```python
from build123d import *

# Parameters (mm, degrees)
SKETCH1_R           = 6
SKETCH1_R_2         = 4.1
BOSS_EXTRUDE1_DEPTH = 5
SKETCH7_R           = 2.6
CUT_EXTRUDE1_DEPTH  = 7
BOSS_EXTRUDE7_DEPTH = 8
SKETCH9_R           = 1.6
CUT_EXTRUDE2_DEPTH  = 7
CUT_EXTRUDE3_DEPTH  = 10
SKETCH11_R          = 1
CUT_EXTRUDE4_DEPTH  = 10


with BuildPart() as part:
    # Sketch1 → Boss-Extrude1 (new body)
    with BuildSketch(Plane.XY):
        with BuildLine():
            Line((-58.265804598, 27.46480771), (50.206034483, 32.957769253))
            ThreePointArc((50.206034483, 32.957769253), (84.875, 0), (50.206034483, -32.957769253))
            Line((50.206034483, -32.957769253), (-58.265804598, -27.46480771))
            ThreePointArc((-58.265804598, -27.46480771), (-61.107119662, -27.172397082), (-63.902777778, -26.586845234))
            Line((-63.902777778, -26.586845234), (-105.963888889, -15.468709954))
            ThreePointArc((-105.963888889, -15.468709954), (-117.875, 0), (-105.963888889, 15.468709954))
            Line((-105.963888889, 15.468709954), (-63.902777778, 26.586845234))
            ThreePointArc((-63.902777778, 26.586845234), (-61.107119662, 27.172397082), (-58.265804598, 27.46480771))
        make_face()
        with Locations((51.875, 0)):
            Circle(SKETCH1_R, mode=Mode.SUBTRACT)
        with Locations((-101.875, 0)):
            Circle(SKETCH1_R_2, mode=Mode.SUBTRACT)
        with BuildLine():
            Line((-46.875, -18.2), (-56.875, -18.2))
            ThreePointArc((-56.875, -18.2), (-75.075, 0), (-56.875, 18.2))
            Line((-56.875, 18.2), (-46.875, 18.2))
            ThreePointArc((-46.875, 18.2), (-28.675, 0), (-46.875, -18.2))
        make_face(mode=Mode.SUBTRACT)
    extrude(amount=BOSS_EXTRUDE1_DEPTH)

    # Sketch7 → Cut-Extrude1 (cut)
    with BuildSketch(Plane.XY.offset(5)):
        with Locations((29.375, 0)):
            Circle(SKETCH7_R)
        with Locations((74.375, 0)):
            Circle(SKETCH7_R)
    extrude(amount=-CUT_EXTRUDE1_DEPTH, mode=Mode.SUBTRACT)

    # Sketch8 → Boss-Extrude7 (add)
    with BuildSketch(Plane.XY.offset(5)):
        Polygon((-28.993802154, 25), (-26.684401077, 21), (-22.065598923, 21), (-19.756197846, 25), (-22.065598923, 29), (-26.684401077, 29), align=None)
        Polygon((-25.775, 27.424871131), (-27.175, 25), (-25.775, 22.575128869), (-22.975, 22.575128869), (-21.575, 25), (-22.975, 27.424871131), align=None, mode=Mode.SUBTRACT)
    boss_extrude7 = extrude(amount=-BOSS_EXTRUDE7_DEPTH)

    # Sketch9 → Cut-Extrude2 (cut)
    with BuildSketch(Plane.XY.offset(5)):
        with Locations((-24.375, 25)):
            Circle(SKETCH9_R)
    cut_extrude2 = extrude(amount=-CUT_EXTRUDE2_DEPTH, mode=Mode.SUBTRACT)

    # Mirror1: Boss-Extrude7 across plane
    add(boss_extrude7.mirror(Plane.ZX))

    # Mirror2: Cut-Extrude2 across plane
    add(cut_extrude2.mirror(Plane.ZX), mode=Mode.SUBTRACT)

    # Sketch10 → Cut-Extrude3 (cut)
    with BuildSketch(Plane.XY.offset(5)):
        with BuildLine():
            Line((-80.875, 17), (-74.875, 17))
            ThreePointArc((-74.875, 17), (-72.875, 15), (-74.875, 13))
            Line((-74.875, 13), (-80.875, 13))
            ThreePointArc((-80.875, 13), (-82.875, 15), (-80.875, 17))
        make_face()
        with BuildLine():
            Line((-22.875, 17), (-28.875, 17))
            ThreePointArc((-28.875, 17), (-30.875, 15), (-28.875, 13))
            Line((-28.875, 13), (-22.875, 13))
            ThreePointArc((-22.875, 13), (-20.875, 15), (-22.875, 17))
        make_face()
        with BuildLine():
            Line((-22.875, -17), (-28.875, -17))
            ThreePointArc((-28.875, -17), (-30.875, -15), (-28.875, -13))
            Line((-28.875, -13), (-22.875, -13))
            ThreePointArc((-22.875, -13), (-20.875, -15), (-22.875, -17))
        make_face()
        with BuildLine():
            Line((-80.875, -17), (-74.875, -17))
            ThreePointArc((-74.875, -17), (-72.875, -15), (-74.875, -13))
            Line((-74.875, -13), (-80.875, -13))
            ThreePointArc((-80.875, -13), (-82.875, -15), (-80.875, -17))
        make_face()
    extrude(amount=-CUT_EXTRUDE3_DEPTH, mode=Mode.SUBTRACT)

    # Sketch11 → Cut-Extrude4 (cut)
    with BuildSketch(Plane.XY.offset(5)):
        with Locations((-115.168208365, -3.514699328)):
            Circle(SKETCH11_R)
        with Locations((-88.581791635, 3.514699328)):
            Circle(SKETCH11_R)
    extrude(amount=-CUT_EXTRUDE4_DEPTH, mode=Mode.SUBTRACT)


solid = part.part
```
For this review, take the finished solid that the model builds, in its own axes (mm). A direction names the side the tool comes from. Give positions to 0.01 mm unless a question says otherwise; leave off trailing zeros. Write each loop counter-clockwise with the first axis right and the second up, starting at its lowest first coordinate (ties: lowest second). Pieces come first, ordered by that corner, then holes. Notation, with made-up numbers: M 5,-1 L 28,-1 A30 cw 28,22 Z; hole C -12,-12.75 d8. An arc over 180 degrees is marked long. Answer as a JSON object with one key per item and string values. Group by question number.
Item 1: Consider section D-D on x = 43.5. Write out the cut boundary in (y, z), plus the area to 3 significant figures.
Item 2: Consider section A-A on y = 0. Write out the cut boundary in (x, z) (3 decimals), plus the area to 3 significant figures.
Item 3: For probe 1 along Z at (x, y) = (23, 29.5); probe 2 along Y at (x, z) = (-76.5, 2.75); probe 3 along X at (y, z) = (7, 2.25) (1 decimal), list the stretches that pass through material, from the lowest coordinate up. Write a range as [from, to].
Item 4: Draft analysis for pull direction Y (two halves, no side actions). For faces 1 (the flat face through (-22, 27, -3)), 2 (the cylindrical face through (-117.872, -0.294, 2.465)), 3 (the flat face through (-26, 17, 3)), 4 (the flat face through (-84.639, -21.106, 2.465)), state which applies: +Y half, -Y half, draft (parallel to the pull), parting line (faces both ways), or undercut.
Item 5: Consider section B-B on x = -51. Write out the cut boundary in (y, z), plus the area to 3 significant figures.
Item 6: For pin 1 Ø9.5 at (x, y) = (-101.875, 0) entering from +Z; pin 2 Ø15.5 at (x, y) = (51.875, 0) entering from -Z; pin 3 Ø2.5 at (x, z) = (-77.5, 1.5) entering from -Y; pin 4 Ø3.5 at (x, z) = (-24.5, -2) entering from +Y, all flat-tipped, find the tip position at first contact; note any pin that passes through.
Item 7: Consider section C-C on z = 2.5. Count the separate pieces of the cut face and the enclosed holes in it, plus the area to 3 significant figures.
Item 8: Tool access review of faces 5 (the flat face through (-78, 17, 3)), 6 (the flat face through (5, 0, 5)), 7 (the flat face through (-26, 26, 0)): name each direction out of +Z, -Z, +X, -X, +Y, -Y from which nothing blocks a thin tool from reaching the whole face with its end or side.
Check result:
{
 "1": {"outline": "M -32.62,0 L 32.62,0 L 32.62,5 L -32.62,5 Z", "area": "326 mm^2"},
 "2": {"outline": "M -117.875,0 L -105.975,0 L -105.975,5 L -117.875,5 Z; M -97.775,0 L -75.075,0 L -75.075,5 L -97.775,5 Z; M -28.675,0 L 26.775,0 L 26.775,5 L -28.675,5 Z; M 31.975,0 L 45.875,0 L 45.875,5 L 31.975,5 Z; M 57.875,0 L 71.775,0 L 71.775,5 L 57.875,5 Z; M 76.975,0 L 84.875,0 L 84.875,5 L 76.975,5 Z", "area": "629 mm^2"},
 "3": {"probe 1": "z = [0, 5]", "probe 2": "y = [-23.26, -17], [-13, 13], [17, 23.26]", "probe 3": "x = [-116.3, -73.7], [-30.1, 84.1]"},
 "4": {"face 1": "draft", "face 2": "parting line", "face 3": "undercut", "face 4": "-Y half"},
 "5": {"outline": "M -27.83,0 L -18.2,0 L -18.2,5 L -27.83,5 Z; M 18.2,0 L 27.83,0 L 27.83,5 L 18.2,5 Z", "area": "96.3 mm^2"},
 "6": {"pin 1": "stops at z = 5", "pin 2": "stops at z = 0", "pin 3": "stops at y = -23.32", "pin 4": "stops at y = 29"},
 "7": {"separate pieces": "1", "enclosed holes": "13", "area": "8,940 mm^2"},
 "8": {"face 5": "+Z, -Z", "face 6": "+Z, +X, -X, +Y, -Y", "face 7": "-Z"}
}
